Model file for the job. Use its own axes, mm. A direction names the side the tool comes from. Give positions to 0.01 mm unless a question says otherwise; leave off trailing zeros. Loops run counter-clockwise (first coordinate to the right, second up) from the corner with the lowest first, then second, coordinate; pieces in that order, holes last. Notation, with made-up numbers: M 16,58.5 L 23,58.5 A17 ccw 23,89.5 Z; hole C -11.75,31.5 d6. An arc over 180 degrees is marked long. Answer in a Markdown table with one row per item.
Autodesk Inventor part; units mm, degrees
ref_plane "YZ Plane" through (0, 0, 0) normal (1, 0, 0) x (0, 1, 0)
ref_plane "XZ Plane" through (0, 0, 0) normal (0, 1, 0) x (-1, 0, 0)
ref_plane "XY Plane" through (0, 0, 0) normal (0, 0, 1) x (1, 0, 0)
sketch "Sketch1" plane through (0, 0, 0) normal (0, 0, 1) x (1, 0, 0)
  line L0 (-7.72, -6.385) -> (7.72, -6.385)
  line L1 (7.72, -6.385) -> (5.4683, 6.385)
  line L2 (5.4683, 6.385) -> (-5.4683, 6.385)
  line L3 (-5.4683, 6.385) -> (-7.72, -6.385)
  point P0 (0, 0)
  point P1 (0, -6.385)
  point P2 (-6.5942, 0)
  dimension "d0" = 15.44
  dimension "d1" = 80
  dimension "d2" = 12.77
extrude "Extrusion1" add sketch "Sketch1" along normal mid plane 8
sketch "Sketch2" plane through (-7.72, -6.385, 4) normal (0, -1, 0) x (1, 0, 0)
  line L0 (15.44, -8) -> (15.44, 0)
  line L1 (3.72, -4) -> (11.72, -4) construction
  circle A0 centre (3.72, -4) radius 2.5
  circle A1 centre (11.72, -4) radius 2.5
  point P0 (7.72, -4)
  point P1 (7.72, -4)
  dimension "d5" = 5
  dimension "d6" = 8
extrude "Extrusion2" cut sketch "Sketch2" against normal blind 6
sketch "Sketch3" plane through (-5.4683, 6.385, 4) normal (0, 1, 0) x (1, 0, 0)
  circle A0 centre (5.4683, 4) radius 2.44
  dimension "d9" = 4.88
extrude "Extrusion3" add sketch "Sketch3" along normal blind 2
fillet "Fillet1" radius 0.4 1 edges at (-2.44, 8.385, 0)
fillet "Fillet2" radius 0.75 4 edges at (-6.5942, 0, 4) (-6.5942, 0, -4) (6.5942, 0, -4) (6.5942, 0, 4)
fillet "Fillet3" radius 0.75 8 edges at (-5.2452, 6.385, -3.7803) (-5.4683, 6.385, 0) (-5.2452, 6.385, 3.7803) (0, 6.385, 4) (5.2452, 6.385, 3.7803) (5.4683, 6.385, 0) (5.2452, 6.385, -3.7803) (0, 6.385, -4)
sketch "Sketch4" plane through (-7.72, -6.385, -3.25) normal (-0.9848, 0.1736, 0) x (0, 0, 1)
  line L0 (6.5, 0) -> (0, 0)
  circle A0 centre (3.25, 9.5) radius 2
  point P0 (3.25, 7.6286)
  dimension "d15" = 4
  dimension "d16" = 9.5
extrude "Extrusion4" cut sketch "Sketch4" against normal blind 2
mirror "Mirror1" about plane through (0, 0, 0) normal (1, 0, 0) of "Extrusion4"
properties part number "TORSO" material "250"
Q1. Probe probe 1 along Z at (x, y) = (4, -3.8); probe 2 along X at (y, z) = (-5, 2); probe 3 along X at (y, z) = (-2, 1.5). List the from-to ranges inside material, lowest first.
Reported:
| item | result |
|---|---|
| probe 1 | -4 to -2.5, 2.5 to 4 |
| probe 2 | -7.48 to -5.5, -2.5 to 2.5, 5.5 to 7.48 |
| probe 3 | -6.95 to -6, -2 to 2, 6 to 6.95 |
Q2. Saw through at C-C (y = -1.25). Give the number of separate pieces and of enclosed holes in the cut face, and give its area (3 significant figures).
Reported:
| item | result |
|---|---|
| separate pieces | 1 |
| enclosed holes | 2 |
| area | 69.3 mm² |
Q3. Mould opens along Z. For faces 1 (the face through (6.664, -0.395, -0.046)), 2 (the face through (-1.615, -3.427, 0.751)), 3 (the face through (0, 0, 4)), 4 (the face through (0, 0, -4)) say: released by +Z, released by -Z, zero draft, split by the parting line, or undercut.
Reported:
| item | result |
|---|---|
| face 1 | zero draft |
| face 2 | undercut |
| face 3 | released by +Z |
| face 4 | released by -Z |
Q4. Saw through at A-A (x = 0). Give the cut face in (y, z) (3 decimals), and give its area (3 significant figures).
Reported:
| item | result |
|---|---|
| outline | M -6.385,-4 L 5.635,-4 A0.75 ccw 6.385,-3.25 L 6.385,-2.44 L 7.985,-2.44 A0.4 ccw 8.385,-2.04 L 8.385,2.04 A0.4 ccw 7.985,2.44 L 6.385,2.44 L 6.385,3.25 A0.75 ccw 5.635,4 L -6.385,4 Z |
| area | 112 mm² |
Q5. Saw through at D-D (x = 3.5). Give the cut face in (y, z) (3 decimals).
Reported:
| item | result |
|---|---|
| outline | M -6.385,-4 L 5.635,-4 A0.75 ccw 6.385,-3.25 L 6.385,3.25 A0.75 ccw 5.635,4 L -6.385,4 L -6.385,2.449 L -0.385,2.449 L -0.385,-2.449 L -6.385,-2.449 Z |
Q6. 3-axis set-ups, long thin cutter, end or side, ignore diameter. For faces 5 (the face through (2.2, 6.385, -1.5)), 6 (the face through (4, -0.385, 0)), 7 (the face through (4.094, 2.651, 0.028)): which of +Z, -Z, +X, -X, +Y, -Y reach the whole face in a straight line?
Reported:
| item | result |
|---|---|
| face 5 | +Y |
| face 6 | -Y |
| face 7 | none |
Q7. Saw through at B-B (z = -2.75). Give the cut face in (x, y) (3 decimals).
Reported:
| item | result |
|---|---|
| outline | M -7.72,-6.385 L 7.72,-6.385 L 5.578,5.765 A0.75 ccw 4.839,6.385 L -4.839,6.385 A0.75 ccw -5.578,5.765 Z |
Q8. Drop flat-ended pins along their axis: pin 1 (1 mm diameter, centred on x = -3.5, z = -3, fed in from +Y) (3 decimals); pin 2 (4 mm diameter, centred on y = -1.5, z = 0.5, fed in from -X). Give the stop position or say it passes through.
Reported:
| item | result |
|---|---|
| pin 1 | y = 6.385 |
| pin 2 | x = -7.21 |
